Geometry: final body of the model. Coordinates: model frame, mm. Face numbers are marked on the shaded views. Give positions to 0.01 mm unless a question says otherwise; leave off trailing zeros. Write each loop counter-clockwise with the first axis right and the second up, starting at its lowest first coordinate (ties: lowest second). Pieces come first, ordered by that corner, then holes.
Q1. Draft query along Z for the marked faces 1 and 2. Return one class per face: pulls with the +Z half, pulls with the -Z half, needs draft (parallel to the pull), parting line crosses it, or undercut.
Q2. Cut plane A-A on x = 47. Return the cut outline in (y, z).
Q3. Cut plane B-B on z = -17. Return the cut outline in (x, y).
Q4. Pin query (flat end, axial travel): pin 1 (8 mm diameter, centred on x = -21, z = 32.5, fed in from +Y); pin 2 (1.5 mm diameter, centred on y = 2, z = -37, fed in from +X); pin 3 (1.5 mm diameter, centred on y = 1, z = -37.5, fed in from -X); pin 4 (0.9 mm diameter, centred on x = 18.5, y = 1.5, fed in from -Z). Return the tip coordinate at first contact, or that it passes through.
Q5. Cut plane C-C on x = -45. Return the cut outline in (y, z), plus the area to 3 significant figures.
Q6. Line query: L1, parallel to X at y = 2.15, z = -36; L2, parallel to X at y = 1.65, z = 8.5; L3, parallel to Z at x = -19, y = 2.65. Output: solid intervals per line, ascending.
```python
from build123d import *

# Parameters (mm, degrees)
BOSS_EXTRUDE6_DEPTH   = 3
BOSS_EXTRUDE6_2_DEPTH = 3
SKETCH4_W             = 119.7
SKETCH4_H             = 55
BOSS_EXTRUDE7_DEPTH   = 1
FILLET13_R            = 3
FILLET14_R            = 1
FILLET15_R            = 1
FILLET16_R            = 3
FILLET17_R            = 3
FILLET18_R            = 1
FILLET19_R            = 3
FILLET20_R            = 1


with BuildPart() as part:
    # Sketch3 → Boss-Extrude6 (new body)
    with BuildSketch(Plane(origin=(0, 0, 0), x_dir=(1, 0, 0), z_dir=(0, 1, 0))):
        Polygon((-55.6, -27.5), (-59.85, -27.5), (-59.85, 27.5), (-55.6, 27.5), (-55.6, 42.5), (-57.6, 42.5), (-57.6, 30.5), (-62.85, 30.5), (-62.85, -30.5), (-57.6, -30.5), (-57.6, -42.5), (-55.6, -42.5), align=None)
    extrude(amount=BOSS_EXTRUDE6_DEPTH)



with BuildPart() as body_2:
    # Sketch3 → Boss-Extrude6 2 (new body)
    with BuildSketch(Plane(origin=(0, 0, 0), x_dir=(1, 0, 0), z_dir=(0, 1, 0))):
        Polygon((59.85, -27.5), (-24.4, -27.5), (-24.4, -42.5), (-22.4, -42.5), (-22.4, -30.5), (62.85, -30.5), (62.85, 30.5), (-22.4, 30.5), (-22.4, 42.5), (-24.4, 42.5), (-24.4, 27.5), (59.85, 27.5), align=None)
    extrude(amount=BOSS_EXTRUDE6_2_DEPTH)


with BuildPart() as part_1:
    add(part.part)

    add(body_2.part)  # Boss-Extrude7 merges body 2
    # Sketch4 → Boss-Extrude7 (add)
    with BuildSketch(Plane(origin=(0, 0, 0), x_dir=(1, 0, 0), z_dir=(0, 1, 0))):
        Rectangle(SKETCH4_W, SKETCH4_H)
    extrude(amount=BOSS_EXTRUDE7_DEPTH)

    # Fillet13
    fillet13_edges = [part_1.edges().sort_by_distance(p)[0] for p in [
        (-62.85, 1.5, 30.5),
        (-62.85, 1.5, -30.5),
        (62.85, 1.5, 30.5),
        (62.85, 1.5, -30.5),
    ]]
    fillet(fillet13_edges, radius=FILLET13_R)

    # Fillet14
    fillet14_edges = [part_1.edges().sort_by_distance(p)[0] for p in [
        (-59.85, 2, -27.5),
        (-59.85, 2, 27.5),
        (59.85, 2, -27.5),
        (59.85, 2, 27.5),
    ]]
    fillet(fillet14_edges, radius=FILLET14_R)

    # Fillet15
    fillet15_edges = [part_1.edges().sort_by_distance(p)[0] for p in [
        (-22.4, 1.5, 42.5),
        (-24.4, 1.5, 42.5),
        (-55.6, 1.5, 42.5),
        (-57.6, 1.5, 42.5),
        (-55.6, 1.5, -42.5),
        (-57.6, 1.5, -42.5),
        (-22.4, 1.5, -42.5),
        (-24.4, 1.5, -42.5),
    ]]
    fillet(fillet15_edges, radius=FILLET15_R - 0.0001)  # a hair under: the kernel refuses the full size

    # Fillet16
    fillet16_edges = [part_1.edges().sort_by_distance(p)[0] for p in [
        (-22.4, 1.5, -30.5),
        (-57.6, 1.5, -30.5),
        (-57.6, 1.5, 30.5),
        (-22.4, 1.5, 30.5),
    ]]
    fillet(fillet16_edges, radius=FILLET16_R)

    # Fillet17
    fillet17_edges = [part_1.edges().sort_by_distance(p)[0] for p in [
        (-55.6, 2, -27.5),
        (-24.4, 2, -27.5),
    ]]
    fillet(fillet17_edges, radius=FILLET17_R)

    # Fillet18
    fillet18_edges = [part_1.edges().sort_by_distance(p)[0] for p in [
        (-55.6, 0.5, -27.5),
        (-24.4, 0.5, -27.5),
    ]]
    fillet(fillet18_edges, radius=FILLET18_R)

    # Fillet19
    fillet19_edges = [part_1.edges().sort_by_distance(p)[0] for p in [
        (-55.6, 2, 27.5),
        (-24.4, 2, 27.5),
    ]]
    fillet(fillet19_edges, radius=FILLET19_R)

    # Fillet20
    fillet20_edges = [part_1.edges().sort_by_distance(p)[0] for p in [
        (-55.6, 0.5, 27.5),
        (-24.4, 0.5, 27.5),
    ]]
    fillet(fillet20_edges, radius=FILLET20_R)


solid = part_1.part
```
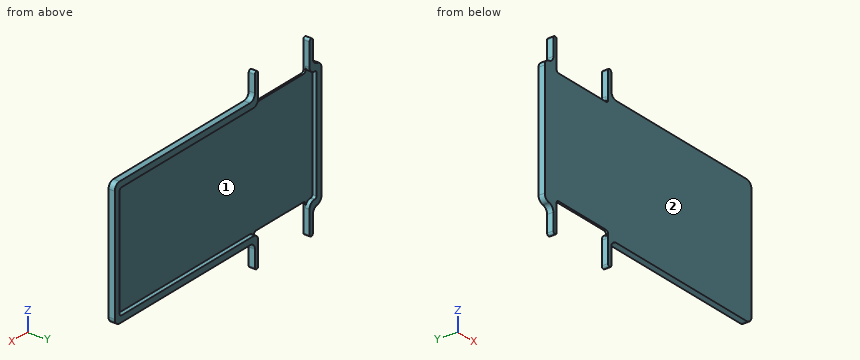
Data:
1. face 1: undercut
1. face 2: needs draft
2. outline: (0, -30.5) - (3, -30.5) - (3, -27.5) - (1, -27.5) - (1, 27.5) - (3, 27.5) - (3, 30.5) - (0, 30.5) - close
3. outline: (-62.85, 0) - (62.85, 0) - (62.85, 3) - (59.85, 3) - (59.85, 1) - (-59.85, 1) - (-59.85, 3) - (-62.85, 3) - close
4. pin 1: stops at y = 3
4. pin 2: stops at x = -22.4
4. pin 3: stops at x = -57.6
4. pin 4: stops at z = -30.5
5. outline: (0, -27.5) - (1, -27.5) - (1, 27.5) - (0, 27.5) - close
5. area: 55.0 mm2
6. L1: x = -57.6 to -55.6, -24.4 to -22.4
6. L2: x = -62.85 to -59.85, 59.85 to 62.85
6. L3: z = -30.5 to -27.5, 27.5 to 30.5
